For this review, take the finished solid that the model builds, in its own axes (mm). Coordinates: 2 decimals unless noted, no trailing zeros. Write each loop counter-clockwise with the first axis right and the second up, starting at its lowest first coordinate (ties: lowest second). Pieces come first, ordered by that corner, then holes. Notation, with made-up numbers: (56, 18) - (65, 18) arc R34 ccw to (65, 50) - close; hole circle Ø8 at (11, 22). An arc over 180 degrees is marked (long way). Write each question's results on one line, items separated by ' | '.
from build123d import *

# Parameters (mm, degrees)
SKETCH1_W            = 698
SKETCH1_H            = 485.9
BOSS_EXTRUDE1_DEPTH  = 5
FILLET1_R            = 40
M6_TAPPED_HOLE1_D    = 5
M6_TAPPED_HOLE2_D    = 5
M4_TAPPED_HOLE1_D    = 3.3
SKETCH8_W            = 286.7
SKETCH8_H            = 199.7
CUT_EXTRUDE1_DEPTH   = 6
FILLET2_R            = 10
M4_CLEARANCE_HOLE1_D = 4.5


with BuildPart() as part:
    # Sketch1 → Boss-Extrude1 (new body)
    with BuildSketch(Plane.XY):
        Rectangle(SKETCH1_W, SKETCH1_H)
    extrude(amount=BOSS_EXTRUDE1_DEPTH)

    # Fillet1
    fillet1_edges = [part.edges().sort_by_distance(p)[0] for p in [
        (-349, 242.95, 2.5),
        (349, 242.95, 2.5),
        (349, -242.95, 2.5),
        (-349, -242.95, 2.5),
    ]]
    fillet(fillet1_edges, radius=FILLET1_R)

    # M6 Tapped Hole1 (through all)
    with Locations(Plane.XY.offset(5)):
        with Locations((-333, 153.95), (-333, 123.95), (-333, 93.95)):
            m6_tapped_hole1 = Hole(M6_TAPPED_HOLE1_D / 2)

    # M6 Tapped Hole2 (through all)
    with Locations(Plane.XY.offset(5)):
        with Locations((314, 25), (289, 0), (314, -25)):
            Hole(M6_TAPPED_HOLE2_D / 2)

    # Mirror1: M6 Tapped Hole1 across plane
    add(m6_tapped_hole1.mirror(Plane.ZX), mode=Mode.SUBTRACT)

    # M4 Tapped Hole1 (through all)
    with Locations(Plane.XY.offset(5)):
        with Locations((328.180642757, 175.458967428), (328.180642757, 139.458967428)):
            Hole(M4_TAPPED_HOLE1_D / 2)

    # Sketch8 → Cut-Extrude1 (cut, through all)
    with BuildSketch(Plane.XY.offset(5)):
        Rectangle(SKETCH8_W, SKETCH8_H)
    extrude(amount=-CUT_EXTRUDE1_DEPTH, mode=Mode.SUBTRACT)

    # Fillet2
    fillet2_edges = [part.edges().sort_by_distance(p)[0] for p in [
        (143.35, -99.85, 2.5),
        (-143.35, -99.85, 2.5),
        (-143.35, 99.85, 2.5),
        (143.35, 99.85, 2.5),
    ]]
    fillet(fillet2_edges, radius=FILLET2_R)

    # M4 Clearance Hole1 (through all)
    with Locations(Plane.XY.offset(5)):
        with Locations((152.5, 90.1), (152.5, 45.05), (133.6, 109), (66.8, 109), (0, 109), (-66.8, 109), (-133.6, 109), (-152.5, 90.1), (-152.5, 45.05), (-152.5, 0), (-152.5, -45.05), (-152.5, -90.1), (-133.6, -109), (-66.8, -109), (0, -109), (66.8, -109), (133.6, -109), (152.5, -90.1), (152.5, -45.05), (152.5, 0)):
            Hole(M4_CLEARANCE_HOLE1_D / 2)


solid = part.part
Q1. Take a section at A-A on x = 93. State the section outline as (y, z) points.
Results found:
outline: (-242.95, 0) - (-99.85, 0) - (-99.85, 5) - (-242.95, 5) - close; (99.85, 0) - (242.95, 0) - (242.95, 5) - (99.85, 5) - close
Q2. Wall thickness on line 1 along X through (y, z) = (-0.5, 3.7); line 2 along X through (y, z) = (-6, 0.45); line 3 along Y through (x, z) = (-112, 2.05): over which ranges is each line inside the solid? List them lowest first. Write a range as from..to.
Results found:
line 1: -349..-154.69, -150.31..-143.35, 143.35..150.31, 154.69..286.55, 291.45..349 | line 2: -349..-143.35, 143.35..349 | line 3: -242.95..-99.85, 99.85..242.95
Q3. Take a section at B-B on z = 3.3. State how many separate pieces and enclosed holes the cut face has, plus the area to 3 significant figures.
Results found:
separate pieces: 1 | enclosed holes: 32 | area: 280,000 mm2
Q4. For pin 1 (4 mm diameter, centred on x = -152.5, y = 45.05, fed in from +Z), flat-tipped, find the tip position at first contact; note if it passes through.
Results found:
pin 1: through
